Could you check a few things on this model? Use its own coordinates, in mm. Round coordinates to 2 decimals unless told otherwise and drop trailing zeros. Loops run counter-clockwise (first coordinate to the right, second up) from the corner with the lowest first, then second, coordinate; pieces in that order, holes last. Notation, with made-up numbers: (63.5, -14.5) -> (72.5, -14.5) arc R5 cw to (72.5, -8.5) -> close; hole circle Ø1 at (10, 34.5). An arc over 180 degrees is marked (long way). One line per item, written item: value.
Autodesk Inventor part; units mm, degrees
ref_plane "YZ Plane" through (0, 0, 0) normal (1, 0, 0) x (0, 1, 0)
ref_plane "XZ Plane" through (0, 0, 0) normal (0, 1, 0) x (-1, 0, 0)
ref_plane "XY Plane" through (0, 0, 0) normal (0, 0, 1) x (1, 0, 0)
sketch "Sketch1" plane through (0, 0, 0) normal (0, 0, 1) x (1, 0, 0)
  line L0 (0, 0) -> (620, 0)
  line L1 (620, 0) -> (620, 620)
  line L2 (620, 620) -> (0, 620)
  line L3 (0, 620) -> (0, 0)
  line L4 (203, 491) -> (417, 491)
  line L5 (417, 491) -> (417, 377)
  line L6 (417, 377) -> (203, 377)
  line L7 (203, 377) -> (203, 491)
  point P0 (310, 491)
  point P1 (310, 620)
  dimension "d0" = 620
  dimension "d1" = 620
  dimension "d2" = 214
  dimension "d3" = 114
  dimension "d4" = 129
extrude "Extrusion1" add sketch "Sketch1" along normal blind 10
sketch "Sketch2" plane through (0, 0, 10) normal (0, 0, 1) x (1, 0, 0)
  line L0 (0, 0) -> (310, 0)
  line L1 (310, 0) -> (310, 435)
  line L2 (310, 435) -> (0, 435)
  line L3 (0, 435) -> (0, 0)
  line L4 (620, 620) -> (0, 620)
  line L5 (0, 435) -> (620, 435)
  line L6 (620, 435) -> (620, 620)
  line L7 (620, 620) -> (0, 620)
  line L8 (0, 620) -> (0, 435)
  line L9 (310, 435) -> (620, 435)
  line L10 (620, 435) -> (620, 0)
  line L11 (620, 0) -> (310, 0)
  line L12 (310, 0) -> (310, 435)
  line L13 (0, 435) -> (310, 435)
  line L14 (310, 435) -> (310, 620)
  line L15 (310, 620) -> (0, 620)
  line L16 (0, 620) -> (0, 435)
  dimension "d7" = 435
extrude "Extrusion2" cut sketch "Sketch2" against normal through all contours L3 L2 L1 L0 | L1 L5 L10 L11 | L8 L4 L14 L2
sketch "Sketch6" plane through (0, 0, 10) normal (0, 0, 1) x (1, 0, 0)
  line L0 (310, 491) -> (310, 620)
  line L1 (310, 605) -> (296, 605)
  line L2 (296, 605) -> (296, 506)
  line L3 (296, 506) -> (310, 506)
  line L4 (310, 506) -> (310, 605)
  line L5 (417, 435) -> (620, 435)
  line L6 (444, 435) -> (593, 435)
  line L7 (593, 435) -> (593, 421)
  line L8 (593, 421) -> (444, 421)
  line L9 (444, 421) -> (444, 435)
  circle A0 centre (302.5, 595.5) radius 2.5
  circle A1 centre (302.5, 515.5) radius 2.5
  circle A2 centre (453.5, 427.5) radius 2.5
  circle A3 centre (583.5, 427.5) radius 2.5
  point P0 (0, 0)
  point P1 (310, 555.5)
  point P2 (518.5, 435)
  dimension "d28" = 14
  dimension "d29" = 99
  dimension "d30" = 149
  dimension "d31" = 14
  dimension "d32" = 5
  dimension "d33" = 5
  dimension "d34" = 9.5
  dimension "d35" = 9.5
  dimension "d36" = 7.5
  dimension "d37" = 7.5
  dimension "d38" = 5
  dimension "d39" = 5
  dimension "d40" = 9.5
  dimension "d41" = 9.5
  dimension "d42" = 7.5
  dimension "d43" = 7.5
extrude "Extrusion6" add sketch "Sketch6" against normal blind 5
properties part number "TC001b" material "ABS Plastic"
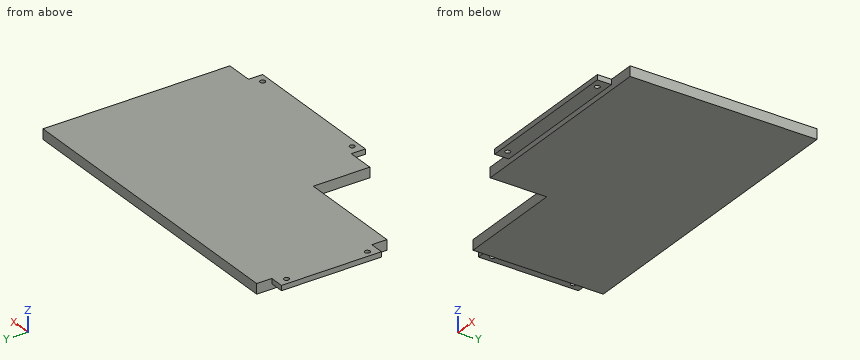
(1) Imagine slicing it at D-D on y = 496.5. Write out the boundary of the cut face in (x, z), then the cut area to 3 significant figures.
Results below:
outline: (310, 0) -> (620, 0) -> (620, 10) -> (310, 10) -> close
area: 3,100 mm²
(2) Imagine slicing it at A-A on z = 6.75. Write out the boundary of the cut face in (x, y), then the cut area to 3 significant figures.
Results below:
outline: (296, 506) -> (310, 506) -> (310, 491) -> (417, 491) -> (417, 435) -> (444, 435) -> (444, 421) -> (593, 421) -> (593, 435) -> (620, 435) -> (620, 620) -> (310, 620) -> (310, 605) -> (296, 605) -> close; hole circle Ø5 at (302.5, 515.5); hole circle Ø5 at (302.5, 595.5); hole circle Ø5 at (453.5, 427.5); hole circle Ø5 at (583.5, 427.5)
area: 54,800 mm²
(3) For pin 1 Ø4.5 at (x, y) = (302.5, 515.5) entering from -Z; pin 2 Ø4 at (x, z) = (304.5, 7) entering from +Y; pin 3 Ø5 at (x, z) = (379.5, 5.5) entering from -Y; pin 4 Ø4 at (x, z) = (304.5, 7.5) entering from -Y, each with a flat end and sliding along its axis, tell me the tip position at first contact or that it passes through.
Results below:
pin 1: passes through
pin 2: stops at y = 605
pin 3: stops at y = 491
pin 4: stops at y = 506
(4) Imagine slicing it at C-C on y = 551. Write out the boundary of the cut face in (x, z), then the cut area to 3 significant figures.
Results below:
outline: (296, 5) -> (310, 5) -> (310, 0) -> (620, 0) -> (620, 10) -> (296, 10) -> close
area: 3,170 mm²
(5) Imagine slicing it at B-B on x = 464.5. Write out the boundary of the cut face in (y, z), then the cut area to 3 significant figures.
Results below:
outline: (421, 5) -> (435, 5) -> (435, 0) -> (620, 0) -> (620, 10) -> (421, 10) -> close
area: 1,920 mm²
(6) Please list where these lines run through material, in increasing order: L1, parallel to X at y = 427.5, z = 7.05; L2, parallel to X at y = 595.5, z = 6.05; L3, parallel to Y at x = 302.5, z = 8.35.
Results below:
L1: x = 444 to 451, 456 to 581, 586 to 593
L2: x = 296 to 300, 305 to 620
L3: y = 506 to 513, 518 to 593, 598 to 605
